For this review, take the finished solid that the model builds, in its own axes (mm). A direction names the side the tool comes from. Round coordinates to 2 decimals unless told otherwise and drop trailing zeros. Order: outer loops, then holes, each group sorted by start corner. A loop starts at its lowest first (then second) coordinate and runs counter-clockwise, first axis right, second up. Notation, with made-up numbers: (-31.5, 63) - (-11.5, 63) arc R32 cw to (-11.5, 91) - close; hole circle Ø7 at (-18.75, 79.5). An arc over 180 degrees is marked (long way). One line per question, with ' | ' between items.
Autodesk Inventor part; units mm, degrees
ref_plane "YZ Plane" through (0, 0, 0) normal (1, 0, 0) x (0, 1, 0)
ref_plane "XZ Plane" through (0, 0, 0) normal (0, 1, 0) x (-1, 0, 0)
ref_plane "XY Plane" through (0, 0, 0) normal (0, 0, 1) x (1, 0, 0)
sketch "Sketch1" plane through (0, 0, 0) normal (0, 1, 0) x (-1, 0, 0)
  arc A0 (172, 0) -> (0, 172) centre (0, 0) ccw
  line L0 (0, 172) -> (0, 0)
  line L1 (172, 0) -> (0, 0)
revolve "Revolution1" add sketch "Sketch1" angle 90 about axis through (0, 0, 172) along (0, 0, -1)
sketch "Sketch2" plane through (-172, 0, 0) normal (0, -1, 0) x (1, 0, 0)
  arc A0 (172, 170) -> (2, 0) centre (172, 0) ccw
  line L0 (172, 0) -> (172, 172)
  line L1 (172, 0) -> (2, 0)
  line L2 (172, 0) -> (172, 170)
revolve "Revolution2" cut sketch "Sketch2" angle 90 about axis through (0, 0, 0) along (0, 0, -1)
sketch "Sketch4" plane through (0, 0, 0) normal (0, -1, 0) x (0.7071068, 0, -0.7071068)
  arc A0 (-120.2082, 120.2082) -> (-120.2082, -120.2082) centre (0, 0) ccw
  line L0 (-170, 0) -> (-150, 0)
  line L1 (-150, 0) -> (-150, -20)
  line L2 (-150, 0) -> (-150, 20)
  line L3 (-150, -20) -> (-170, -20)
  line L4 (-170, -20) -> (-170, 20)
  line L5 (-170, 20) -> (-150, 20)
  dimension "d34" = 20
  dimension "d35" = 20
  dimension "d36" = 20
  dimension "d56" = 20
  dimension "d57" = 40
extrude "Extrusion2" add sketch "Sketch4" against normal blind 60
sketch "Sketch6" plane through (0, 0, 0) normal (1, 0, 0) x (0, -0.7071068, -0.7071068)
  line L0 (-120.2082, 120.2082) -> (0, 0)
  line L1 (-120.2082, -120.2082) -> (-121.6224, -121.6224)
  arc A0 (-121.6224, 121.6224) -> (-121.6224, -121.6224) centre (0, 0) ccw
  line L2 (0, 0) -> (-120.2082, -120.2082)
  arc A1 (-134.3503, 134.3503) -> (-134.3503, -134.3503) centre (0, 0) ccw
  line L3 (-121.6224, 121.6224) -> (-134.3503, 134.3503)
  line L4 (-121.6224, -121.6224) -> (-134.3503, -134.3503)
  point P0 (-74.4097, -74.4097)
revolve "Revolution3" cut sketch "Sketch6" angle 90 about axis through (0, 170, 0) along (0, -1, 0)
sketch "Sketch9" plane through (-120.2082, 0, 91.9239) normal (-0.7071068, 0, -0.7071068) x (-0.7071068, 0, 0.7071068)
  line L0 (0, 0) -> (0, 60)
  line L1 (0, 0) -> (8, 0)
  line L2 (18.8194, 0) -> (0, 0)
  line L3 (8, 0) -> (8, 35)
  line L4 (8, 35) -> (1.5295, 59.1481)
  line L5 (1.5295, 59.1481) -> (4.7087, 60)
  line L6 (0, 60) -> (7.7973, 60)
  line L7 (4.7087, 60) -> (0, 60)
  line L8 (0, 60) -> (0, 0)
  point P0 (-150, 0)
  dimension "d58" = 8
  dimension "d59" = 35
  dimension "d60" = 25
  dimension "d61" = 165
extrude "Extrusion5" cut sketch "Sketch9" against normal blind 40
sketch "Sketch10" plane through (-125.865, 35, 97.5807) normal (0.6830127, -0.258819, -0.6830127) x (-0.7071068, 0, -0.7071068)
  line L0 (0, 25) -> (0, 0)
  line L1 (0, 25) -> (-40, 25)
  line L2 (-40, 0) -> (-40, 25)
  line L3 (-40, 25) -> (0, 25)
  circle A0 centre (-20, 12.5) radius 4
  circle A1 centre (-15.0503, 7.5503) radius 1
  circle A2 centre (-24.9497, 7.5503) radius 1
  circle A3 centre (-24.9497, 17.4497) radius 1
  circle A4 centre (-15.0503, 17.4497) radius 1
  line L4 (-24.9497, 7.5503) -> (-10.9497, 7.5503) construction
  circle A5 centre (-29.8995, 12.5) radius 4
  circle A6 centre (-34.8492, 7.5503) radius 1
  circle A7 centre (-34.8492, 17.4497) radius 1
  line L5 (-15.0503, 17.4497) -> (-1.0503, 17.4497) construction
  line L6 (-15.0503, 7.5503) -> (-1.0503, 7.5503) construction
  circle A8 centre (-10.1005, 12.5) radius 4
  circle A9 centre (-5.1508, 7.5503) radius 1
  circle A10 centre (-5.1508, 17.4497) radius 1
  dimension "d64" = 8
  dimension "d68" = 2
  dimension "d69" = 2
  dimension "d70" = 2
  dimension "d72" = 2
  dimension "d76" = 8
  dimension "d77" = 2
  dimension "d78" = 2
  dimension "d83" = 8
  dimension "d84" = 2
  dimension "d85" = 2
extrude "Extrusion6" cut sketch "Sketch10" against normal blind 3
properties part number "shell" material "Glass"
(1) For probe 1 along Z at (x, y) = (-11, 64.5); probe 2 along Y at (x, z) = (-146.5, 53); probe 3 along Y at (x, z) = (-25, 34), list the stretches that pass through material, from the lowest coordinate up. Write a range as [from, to].
Output values:
probe 1: [156.9, 159.07] | probe 2: [68.03, 72.89] | probe 3: [164.68, 166.74]
(2) Insertion check: pin 1 (8 mm diameter, centred on y = 76.5, z = 113.5, fed in from -X); pin 2 (24.5 mm diameter, centred on x = -103, z = 115.5, fed in from +Y); pin 3 (12 mm diameter, centred on x = -20.5, y = 65, fed in from -Z). Each pin has a flat end and moves straight along its axis. Give the tip position at first contact, or say it passes through.
Output values:
pin 1: x = -109.22 | pin 2: y = 96.31 | pin 3: z = 152.97
(3) For faces 4 (the flat face through (-99.204, 29.58, 127.488)), 5 (the flat face through (-108.454, 59.568, 108.058)), 6 (the flat face through (-127.317, 29.58, 99.033)), list the 3-axis set-ups (+Z, -Z, +X, -X, +Y, -Y) from which the entire face can be reached by the end or side of a thin tool; tool diameter is ignored.
Output values:
face 4: +X, -Y | face 5: -Z, +X | face 6: -Z, -Y
(4) Mouldability with a two-part tool opening along X and no side actions: class faces 1 (the flat face through (-111.921, 17.255, 111.525)), 2 (the flat face through (-111, 0, 118)), 3 (the cylindrical face through (-119.9, 48.6, 100.5)) as released by +X, released by -X, zero draft, split by the parting line, or undercut.
Output values:
face 1: released by +X | face 2: zero draft | face 3: undercut
(5) We need section B-B on z = 30.5. State the section outline as (x, y) points.
Output values:
outline: (-169.27, 0) - (-167.24, 0) arc R167.24 cw to (0, 167.24) - (0, 169.27) arc R169.27 ccw to start
(6) We need section A-A on y = 81. State the section outline as (x, z) points, plus the area to 3 significant figures.
Output values:
outline: (-151.73, 0) - (-149.46, 0) arc R149.46 cw to (0, 149.46) - (0, 151.73) arc R151.73 ccw to start | area: 537 mm^2
